Geometry check sheet. Reference: the model listing, model coordinates, mm. A direction names the side the tool comes from. Coordinates: 2 decimals unless noted, no trailing zeros. Loops run counter-clockwise (first coordinate to the right, second up) from the corner with the lowest first, then second, coordinate; pieces in that order, holes last.
from build123d import *

# Parameters (mm, degrees)
F0_W     = 1.27
F0_H     = 2.2225
F0_W_2   = 7.62
F0_H_2   = 1.5875
F3_DEPTH = 25.4
F6_DEPTH = 6.35


# Not quite as in the source:
# - after a boolean that leaves OpenCascade's solid faulty, fix() repairs it


with BuildPart() as f1:
    # F0 (on Front) → F1 (revolve)
    with BuildSketch(Plane.XZ):
        with Locations((-59.9352485356, 1.11125)):
            Rectangle(F0_W, F0_H)
        with Locations((-59.9352485356, 3.33375)):
            Rectangle(F0_W, F0_H)
        Polygon((-22.4702485356, 5.3975), (-28.8202485356, 5.3975), (-28.8202485356, 3.81), (-28.8202485356, 2.2225), (-22.4702485356, 2.2225), align=None)
        with Locations((-32.6302485356, 3.01625)):
            Rectangle(F0_W_2, F0_H_2)
        Polygon((-36.4402485356, 3.81), (-28.8202485356, 3.81), (-36.4402485356, 5.3975), align=None)
        Polygon((-22.4702485356, -0.9525), (-22.4702485356, 2.2225), (-28.8202485356, 2.2225), (-28.8202485356, 0.635), (-28.8202485356, -0.9525), align=None)
        with Locations((-32.6302485356, 1.42875)):
            Rectangle(F0_W_2, F0_H_2)
        Polygon((-36.4402485356, 2.2225), (-36.4402485356, 3.81), (-36.4402485356, 5.3975), (-38.3452485356, 5.3975), (-38.3452485356, 2.2225), align=None)
        Polygon((-36.4402485356, -0.9525), (-28.8202485356, 0.635), (-36.4402485356, 0.635), align=None)
        Polygon((-36.4402485356, 0.635), (-36.4402485356, 2.2225), (-38.3452485356, 2.2225), (-38.3452485356, -0.9525), (-36.4402485356, -0.9525), align=None)
    revolve(axis=Axis((-41.5202485356, 0, 2.0941267129), (0, 0, 1)))

    add(f1.part.fix(), mode=Mode.REPLACE)

    # F2 (on face) → F3 (cut)
    with BuildSketch(Plane.XY.offset(5.3975)):
        with BuildLine():
            Line((-41.7123280121, 10.8656756712), (-34.9781690591, 8.6776147898))
            Line((-34.9781690591, 8.6776147898), (-33.438209538, 9.7964608733))
            ThreePointArc((-33.438209538, 9.7964608733), (-37.595732707, 12.0784177569), (-42.3005402078, 12.6760066624))
            Line((-42.3005402078, 12.6760066624), (-41.7123280121, 10.8656756712))
        make_face()
        Polygon((-39.8510522546, 5.1372579143), (-34.9781690591, 8.6776147898), (-41.7123280121, 10.8656756712), align=None)
        with BuildLine():
            Line((-51.9134760092, 3.175), (-47.7515368906, 8.9034177569))
            Line((-47.7515368906, 8.9034177569), (-48.3397490863, 10.7137487482))
            ThreePointArc((-48.3397490863, 10.7137487482), (-51.7947643642, 7.4648727041), (-53.8169706598, 3.175))
            Line((-53.8169706598, 3.175), (-51.9134760092, 3.175))
        make_face()
        Polygon((-45.8902611331, 3.175), (-47.7515368906, 8.9034177569), (-51.9134760092, 3.175), align=None)
        with BuildLine():
            Line((-48.3397490863, -10.7137487482), (-47.7515368906, -8.9034177569))
            Line((-47.7515368906, -8.9034177569), (-51.9134760092, -3.175))
            Line((-51.9134760092, -3.175), (-53.8169706598, -3.175))
            ThreePointArc((-53.8169706598, -3.175), (-51.7947643642, -7.4648727041), (-48.3397490863, -10.7137487482))
        make_face()
        Polygon((-51.9134760092, -3.175), (-47.7515368906, -8.9034177569), (-45.8902611331, -3.175), align=None)
        Polygon((-41.7123280121, -10.8656756712), (-34.9781690591, -8.6776147898), (-39.8510522546, -5.1372579143), align=None)
        with BuildLine():
            Line((-33.438209538, -9.7964608733), (-34.9781690591, -8.6776147898))
            Line((-34.9781690591, -8.6776147898), (-41.7123280121, -10.8656756712))
            Line((-41.7123280121, -10.8656756712), (-42.3005402078, -12.6760066624))
            ThreePointArc((-42.3005402078, -12.6760066624), (-37.595732707, -12.0784177569), (-33.438209538, -9.7964608733))
        make_face()
        Polygon((-31.245732707, -3.5403568756), (-31.245732707, 3.5403568756), (-36.1186159026, 0), align=None)
        with BuildLine():
            Line((-29.705773186, 4.659202959), (-31.245732707, 3.5403568756))
            Line((-31.245732707, 3.5403568756), (-31.245732707, -3.5403568756))
            Line((-31.245732707, -3.5403568756), (-29.705773186, -4.659202959))
            ThreePointArc((-29.705773186, -4.659202959), (-29.0435935965, -2.3713037616), (-28.8202485356, 0))
            ThreePointArc((-28.8202485356, 0), (-29.0435935965, 2.3713037616), (-29.705773186, 4.659202959))
        make_face()
    extrude(amount=-F3_DEPTH, mode=Mode.SUBTRACT)

    # F0 (on Front) → F4 (revolve, cut)
    with BuildSketch(Plane.XZ):
        with Locations((-59.9352485356, 3.33375)):
            Rectangle(F0_W, F0_H)
        with Locations((-59.9352485356, 1.11125)):
            Rectangle(F0_W, F0_H)
    revolve(axis=Axis((-41.5202485356, 0, 2.0941267129), (0, 0, 1)), mode=Mode.SUBTRACT)

    add(f1.part.fix(), mode=Mode.REPLACE)

    # F5 (on face) → F6 (join)
    with BuildSketch(Plane.XY.offset(5.3975)):
        with BuildLine():
            Line((-44.6860680874, 0.2412707303), (-42.8942117298, 2.8623155208))
            ThreePointArc((-42.8942117298, 2.8623155208), (-44.1412933261, 1.7918563576), (-44.6860680874, 0.2412707303))
        make_face()
        with BuildLine():
            Line((-43.3121048932, -2.6210447905), (-44.6860680874, 0.2412707303))
            ThreePointArc((-44.6860680874, 0.2412707303), (-44.3825640564, -1.3739631943), (-43.3121048932, -2.6210447905))
        make_face()
        with BuildLine():
            ThreePointArc((-43.3121048932, -2.6210447905), (-41.7615192659, -3.1658195518), (-40.1462853413, -2.8623155208))
            Line((-40.1462853413, -2.8623155208), (-43.3121048932, -2.6210447905))
        make_face()
        with BuildLine():
            ThreePointArc((-40.1462853413, -2.8623155208), (-38.8992037451, -1.7918563576), (-38.3544289838, -0.2412707303))
            Line((-38.3544289838, -0.2412707303), (-40.1462853413, -2.8623155208))
        make_face()
        with BuildLine():
            ThreePointArc((-38.3544289838, -0.2412707303), (-38.3475444778, -0.1207226635), (-38.3452485356, 0))
            ThreePointArc((-38.3452485356, 0), (-38.7122448911, 1.4818031355), (-39.728392178, 2.6210447905))
            Line((-39.728392178, 2.6210447905), (-38.3544289838, -0.2412707303))
        make_face()
        with BuildLine():
            Line((-42.8942117298, 2.8623155208), (-39.728392178, 2.6210447905))
            ThreePointArc((-39.728392178, 2.6210447905), (-41.2789778053, 3.1658195518), (-42.8942117298, 2.8623155208))
        make_face()
    extrude(amount=-F6_DEPTH)


solid = f1.part
(1) Sectioned sample at A-A on z = 2. Record the cut outline in (x, y) (3 decimals).
Findings:
outline: circle Ø35.56 at (-41.52, 0); hole (-53.817, -3.175) arc R12.7 ccw to (-48.34, -10.714) - (-45.89, -3.175) - close; hole (-53.817, 3.175) - (-45.89, 3.175) - (-48.34, 10.714) arc R12.7 ccw to start; hole (-44.686, 0.241) - (-43.312, -2.621) - (-40.146, -2.862) - (-38.354, -0.241) - (-39.728, 2.621) - (-42.894, 2.862) - close; hole (-42.301, -12.676) arc R12.7 ccw to (-33.438, -9.796) - (-39.851, -5.137) - close; hole (-42.301, 12.676) - (-39.851, 5.137) - (-33.438, 9.796) arc R12.7 ccw to start; hole (-36.119, 0) - (-29.706, -4.659) arc R12.7 ccw to (-29.706, 4.659) - close
(2) Sectioned sample at B-B on x = -28. Record the cut outline in (y, z) (1 decimal), and give its area (3 significant figures).
Findings:
outline: (-13.4, -1) - (13.4, -1) - (13.4, 0) - (11.5, 0) - (11.5, 4.4) - (13.4, 4.4) - (13.4, 5.4) - (-13.4, 5.4) - (-13.4, 4.4) - (-11.5, 4.4) - (-11.5, 0) - (-13.4, 0) - close
area: 154 mm2
(3) Draft check along Z on faces 1 (the flat face through (-39, -2, -0.952)), 2 (the flat face through (-33, -16, 0)), 3 (the flat face through (-41.333, 2.743, 2.267)). Enter one of: +Z half, -Z half, draft (parallel to the pull), parting line (faces both ways), or undercut.
Findings:
face 1: -Z half
face 2: undercut
face 3: draft
(4) Sectioned sample at D-D on y = 4. State how many separate pieces and enclosed holes the cut face has, and give its area (3 significant figures).
Findings:
separate pieces: 3
enclosed holes: 0
area: 160 mm2
(5) Sectioned sample at C-C on y = 13.5. Record the cut outline in (x, z) (1 decimal), and give its area (3 significant figures).
Findings:
outline: (-55, -1) - (-28.1, -1) - (-28.1, 0) - (-29.9, 0) - (-29.9, 4.4) - (-28.1, 4.4) - (-28.1, 5.4) - (-55, 5.4) - (-55, 4.4) - (-53.1, 4.4) - (-53.1, 0) - (-55, 0) - close
area: 154 mm2
(6) Gauge pin test, flat ends, axial feed: pin 1 Ø1.5 at (x, z) = (-38, 0) entering from +Y; pin 2 Ø1.5 at (x, y) = (-40, 7) entering from -Z; pin 3 Ø1 at (x, z) = (-39, 2) entering from -Y. Record the tip position at first contact, or that the pin passes through.
Findings:
pin 1: stops at y = 18.85
pin 2: stops at z = -0.67
pin 3: stops at y = -17.66
(7) Access from +Z, -Z, +X, -X, +Y, -Y to the whole of each face (thin tool, end or side, straight path). Record for faces 4 (the conical face through (-36.32, 1.64, 5.32)), 5 (the flat face through (-43.803, 1.533, 2.267)), 6 (the flat face through (-33, -16, 4.445)).
Findings:
face 4: +Z
face 5: +Z, -Z
face 6: none
(8) Scan lines: L1, parallel to Y at x = -50.5, z = 2.75 (3 decimals); L2, parallel to X at y = 8, z = 3.5; L3, parallel to Y at x = -36, z = 1.25. Record each from-to range of solid material in increasing order.
Findings:
L1: y = -15.346 to -8.981, -3.175 to 3.175, 8.981 to 15.346
L2: x = -57.4 to -51.38, -47.46 to -40.78, -35.91 to -25.64
L3: y = -16.9 to -11.44, -7.94 to -0.09, 0.09 to 7.94, 11.44 to 16.9
